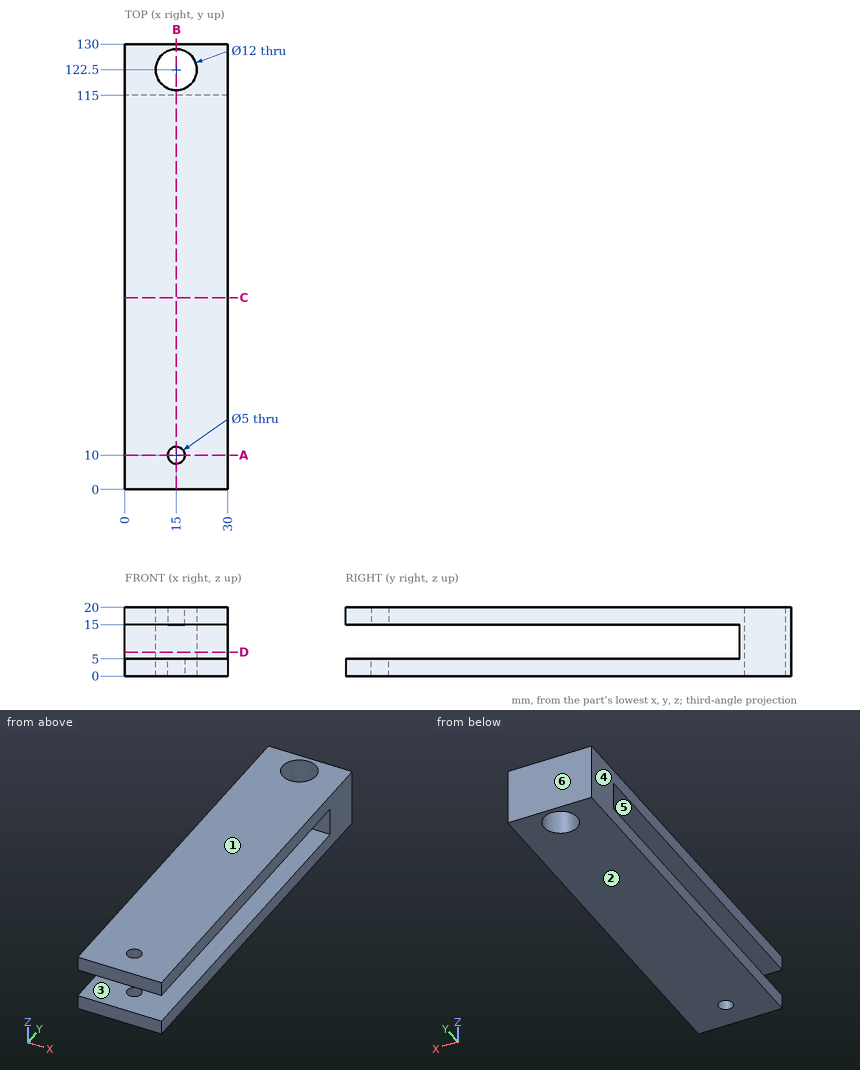
Input: dimensioned drawing with shaded views. Units: mm. Origin: part minimum x, y, z. A direction names the side the tool comes from. Round coordinates to 2 decimals unless told otherwise and drop trailing zeros. Order: outer loops, then holes, each group sorted by start corner. A loop starts at its lowest first (then second) coordinate and runs counter-clockwise, first axis right, second up. Notation, with made-up numbers: (37.25, 48) -> (48.25, 48) arc R21 cw to (48.25, 80) -> close; hole circle Ø6 at (-10, -1). An arc over 180 degrees is marked (long way). One line per item, written item: value. Start each with the question number.
Q1. Pin query (flat end, axial travel): pin 1 (5 mm diameter, centred on x = 18, z = 11.5, fed in from -Y). Return the tip coordinate at first contact, or that it passes through.
Q2. Material intervals for probe 1 along Y at (x, z) = (15, 3.9); probe 2 along Z at (x, y) = (24.5, 58.5); probe 3 along Y at (x, z) = (13.5, 8.25), sorted ascending.
Q3. Draft query along Z for the marked faces 1, 2, 3 and 4. Return one class per face: pulls with the +Z half, pulls with the -Z half, needs draft (parallel to the pull), parting line crosses it, or undercut.
Q4. Section query B-B (x = 15). Return the cut outline in (y, z), plus the area to 3 significant figures.
Q5. Section query A-A (y = 10). Return the cut outline in (x, z).
Q6. Section query D-D (z = 7). Return the cut outline in (x, y).
Q7. Section query C-C (y = 56). Return the cut outline in (x, z).
Q8. Access query for the marked faces 5 and 6. Directions: +Z, -Z, +X, -X, +Y, -Y. A direction counts if a zero-diameter tool reaches every point of the face in a straight line with its end or side. Return the directions, or none.
Findings below:
1. pin 1: y = 115
2. probe 1: 0 to 7.5, 12.5 to 116.5, 128.5 to 130
2. probe 2: 0 to 5, 15 to 20
2. probe 3: 115 to 116.69, 128.31 to 130
3. face 1: pulls with the +Z half
3. face 2: pulls with the -Z half
3. face 3: undercut
3. face 4: needs draft
4. outline: (0, 0) -> (7.5, 0) -> (7.5, 5) -> (0, 5) -> close; (0, 15) -> (7.5, 15) -> (7.5, 20) -> (0, 20) -> close; (12.5, 0) -> (116.5, 0) -> (116.5, 20) -> (12.5, 20) -> (12.5, 15) -> (115, 15) -> (115, 5) -> (12.5, 5) -> close; (128.5, 0) -> (130, 0) -> (130, 20) -> (128.5, 20) -> close
4. area: 1,160 mm²
5. outline: (0, 0) -> (12.5, 0) -> (12.5, 5) -> (0, 5) -> close; (0, 15) -> (12.5, 15) -> (12.5, 20) -> (0, 20) -> close; (17.5, 0) -> (30, 0) -> (30, 5) -> (17.5, 5) -> close; (17.5, 15) -> (30, 15) -> (30, 20) -> (17.5, 20) -> close
6. outline: (0, 115) -> (30, 115) -> (30, 130) -> (0, 130) -> close; hole circle Ø12 at (15, 122.5)
7. outline: (0, 0) -> (30, 0) -> (30, 5) -> (0, 5) -> close; (0, 15) -> (30, 15) -> (30, 20) -> (0, 20) -> close
8. face 5: +X, -X, -Y
8. face 6: +Z, -Z, +X, -X, +Y
